Job drawing, mm, ordinate dimensions from the low corner. One solid piece. Coordinates: 2 decimals unless noted, no trailing zeros. Order: outer loops, then holes, each group sorted by start corner. A loop starts at its lowest first (then second) coordinate and runs counter-clockwise, first axis right, second up. Notation, with made-up numbers: M -37.5,-26.75 L -11.5,-26.75 A26 ccw -11.5,5.25 Z; hole C -13.75,56.5 d2. An arc over 180 degrees is marked long. Write item = value, one per line.
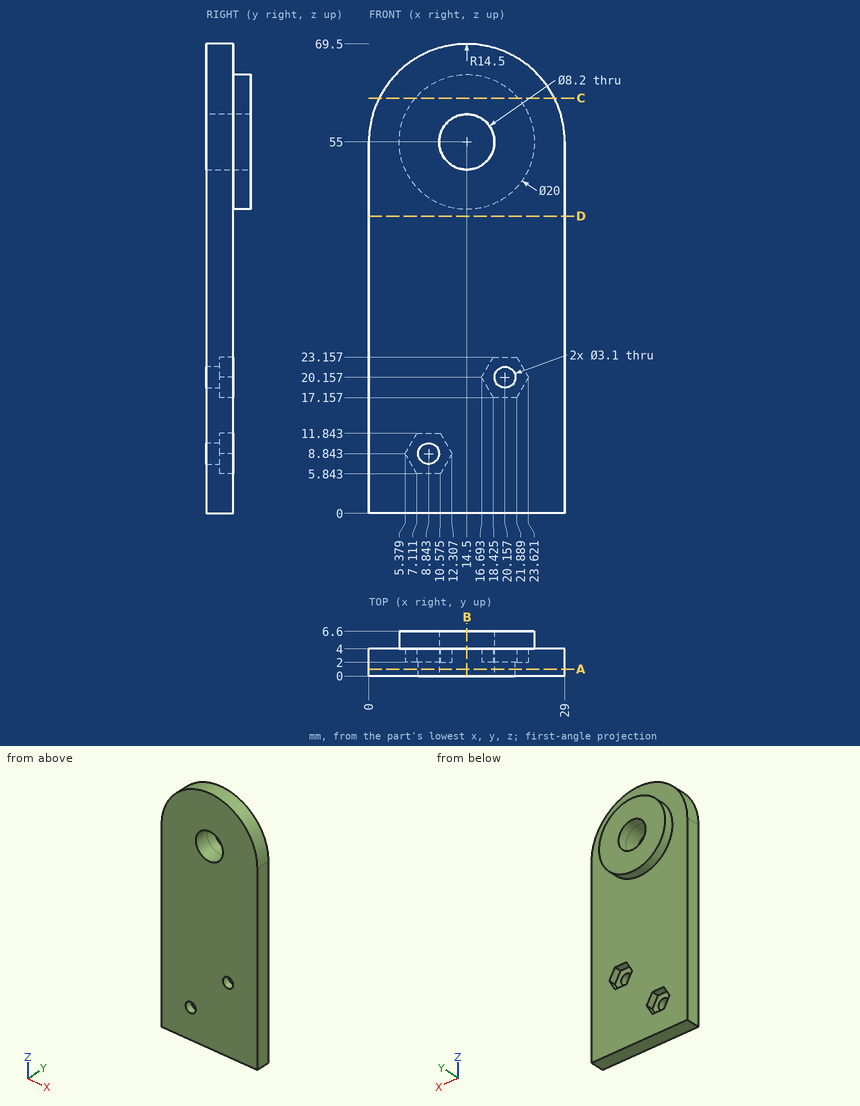
(1) Slice it at D-D, the plane z = 44. Write the cut outline in (x, y).
Evaluation:
outline = M 0,0 L 29,0 L 29,4 L 0,4 Z
(2) Pin check, flat tips, straight feed: pin 1 Ø3 at (x, z) = (10, 10) entering from +Y; pin 2 Ø1.5 at (x, y) = (21, 5.5) entering from -Z; pin 3 Ø1.9 at (x, z) = (8.84, 8.84) entering from +Y; pin 4 Ø1 at (x, y) = (21, 2.5) entering from +Z. Stop position of each tip, or through.
Evaluation:
pin_1 = 4
pin_2 = 46.82
pin_3 = through
pin_4 = 68.2
(3) Slice it at B-B, the plane x = 14.5. Write the cut outline in (y, z).
Evaluation:
outline = M 0,0 L 4,0 L 4,45 L 6.6,45 L 6.6,50.9 L 0,50.9 Z; M 0,59.1 L 6.6,59.1 L 6.6,65 L 4,65 L 4,69.5 L 0,69.5 Z
(4) Slice it at A-A, the plane y = 1. Write the cut outline in (x, z).
Evaluation:
outline = M 0,0 L 29,0 L 29,55 A14.5 ccw 0,55 Z; hole C 8.84,8.84 d3.1; hole C 14.5,55 d8.2; hole C 20.16,20.16 d3.1
(5) Slice it at C-C, the plane z = 61.5. Write the cut outline in (x, y).
Evaluation:
outline = M 1.54,0 L 27.46,0 L 27.46,4 L 22.1,4 L 22.1,6.6 L 6.9,6.6 L 6.9,4 L 1.54,4 Z
(6) Wall check: line 1 (Z direction, x = 14.25, y = 2); line 2 (X direction, y = 5.35, z = 55); line 3 (Y direction, x = 16, z = 39.5). Give the ranges that are in metal, low to high. Write a range as from..to.
Evaluation:
line_1 = 0..50.91, 59.09..69.5
line_2 = 4.5..10.4, 18.6..24.5
line_3 = 0..4
